Input: part model. Units: mm. Frame: model coordinates. Face numbers are marked on the shaded views. A direction names the side the tool comes from. Give positions to 0.01 mm unless a question says otherwise; leave off trailing zeros. Loops run counter-clockwise (first coordinate to the right, second up) from the corner with the lowest first, then second, coordinate; pieces in that order, holes last. Notation, with made-up numbers: M 16.25,-28 L 31.25,-28 A30 ccw 31.25,-3 Z; hole C 12.25,67.5 d3. An arc over 180 degrees is marked long. Use CSV: the item, a comma, the result in double quotes. Start each with the question number.
Q1. Pin query (flat end, axial travel): pin 1 (4 mm diameter, centred on y = -25.5, z = 26.5, fed in from -X); pin 2 (5 mm diameter, centred on y = 29, z = 24, fed in from +X); pin 3 (6.5 mm diameter, centred on x = -4.5, y = 29, fed in from +Z). Return the tip coordinate at first contact, or that it passes through.
Q2. Section B-B, the plane y = 0. Output: boundary loops of the cut face in (x, z), plus the area to 3 significant figures.
Q3. Section A-A, the plane z = 21. Output: boundary loops of the cut face in (x, y).
Q4. Reachability of the marked faces 1, 2, 3, 4 and 5 from +Z, -Z, +X, -X, +Y, -Y: full face, straight path, thin tool, end or side. Return the list, or none.
Q5. Pull-direction query (X, two-part tool) for the marked faces 6, 7 and 8; classes: released by +X, released by -X, zero draft, split by the parting line, or undercut.
Q6. Material intervals for line 1 along Z through (x, y) = (15.5, 8.5); line 2 along X through (y, z) = (18.5, 10); line 3 along X through (y, z) = (-23.5, 17), sorted ascending.
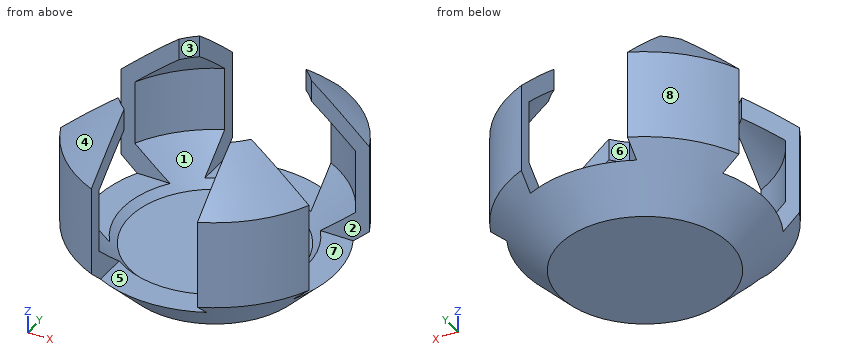
from build123d import *

# Parameters (mm, degrees)
F0_R     = 24
F0_R_2   = 23
F1_DEPTH = 8
F2_DEPTH = 2
F3_W     = 24
F3_H     = 8
F5_W     = 15
F5_H     = 75
F6_DEPTH = 75
F7_W     = 15
F7_H     = 75
F8_DEPTH = 75


with BuildPart() as f1:
    # F0 (on Top) → F1 (new body)
    with BuildSketch(Plane.XY):
        Circle(F0_R)
        Circle(F0_R_2, mode=Mode.SUBTRACT)
    extrude(amount=F1_DEPTH)

    # F0 (on Top) → F2 (join)
    with BuildSketch(Plane.XY):
        Circle(F0_R_2)
    extrude(amount=F2_DEPTH)

    # F3 (on Right) → F4 (revolve)
    with BuildSketch(Plane.YZ):
        with Locations((12, 4)):
            Rectangle(F3_W, F3_H)
        Polygon((24, 8), (24, 0), (38.142136, 14.142136), (38.142136, 39.142136), (24, 53.284271), (24, 47.213203), (34.606602, 36.606602), (34.606602, 18.606602), align=None)
    revolve(axis=Axis((0, 0, 27.5), (0, 0, 1)))

    # F5 (on Right) → F6 (cut, symmetric)
    with BuildSketch(Plane.YZ):
        with Locations((-7.5, 47.5)):
            Rectangle(F5_W, F5_H)
        with Locations((7.5, 47.5)):
            Rectangle(F5_W, F5_H)
    extrude(amount=F6_DEPTH, both=True, mode=Mode.SUBTRACT)

    # F7 (on Front) → F8 (cut, symmetric)
    with BuildSketch(Plane.XZ):
        with Locations((7.5, 47.5)):
            Rectangle(F7_W, F7_H)
        with Locations((-7.5, 47.5)):
            Rectangle(F7_W, F7_H)
    extrude(amount=F8_DEPTH, both=True, mode=Mode.SUBTRACT)


solid = f1.part
A:
1,pin 1,"x = -30.04"
1,pin 2,"x = 27.43"
1,pin 3,"z = 10"
2,outline,"M -34,10 L -24,0 L 24,0 L 34,10 L 26,10 L 24,8 L -24,8 L -26,10 Z"
2,area,"480 mm^2"
3,outline,"M -35.07,-15 A38.14 ccw -15,-35.07 L -15,-31.19 A34.61 cw -31.19,-15 Z; M -35.07,15 L -31.19,15 A34.61 cw -15,31.19 L -15,35.07 A38.14 ccw Z; M 15,-35.07 A38.14 ccw 35.07,-15 L 31.19,-15 A34.61 cw 15,-31.19 Z; M 15,31.19 A34.61 cw 31.19,15 L 35.07,15 A38.14 ccw 15,35.07 Z"
4,face 1,"none"
4,face 2,"+Z, +X, -X"
4,face 3,"+Z"
4,face 4,"+Z, -X, -Y"
4,face 5,"+Z, +Y, -Y"
5,face 6,"undercut"
5,face 7,"zero draft"
5,face 8,"released by -X"
6,line 1,"0 to 8"
6,line 2,"-28.53 to -18.27, 18.27 to 28.53"
6,line 3,"-30.04 to -23.17, 23.17 to 30.04"
